Verification items for the finished model (mm, model axes). Give positions to 0.01 mm unless a question says otherwise; leave off trailing zeros. Write each loop counter-clockwise with the first axis right and the second up, starting at its lowest first coordinate (ties: lowest second). Pieces come first, ordered by that corner, then holes. Notation, with made-up numbers: (65.5, -39) - (93.5, -39) arc R31 ccw to (93.5, -1) - close; hole circle Ø2 at (-21.5, 82.5). An arc over 180 degrees is marked (long way). Put each result on its own line as item: value.
from build123d import *

# Parameters (mm, degrees)
SKETCH1_W           = 355.6
SKETCH1_H           = 406.4
BOSS_EXTRUDE1_DEPTH = 6.35
CUT_EXTRUDE1_DEPTH  = 6.35


with BuildPart() as part:
    # Sketch1 → Boss-Extrude1 (new body)
    with BuildSketch(Plane(origin=(0, 0, 0), x_dir=(1, 0, 0), z_dir=(0, 1, 0))):
        Rectangle(SKETCH1_W, SKETCH1_H)
    extrude(amount=BOSS_EXTRUDE1_DEPTH)

    # Sketch2 → Cut-Extrude1 (cut)
    with BuildSketch(Plane(origin=(0, 6.35, 0), x_dir=(1, 0, 0), z_dir=(0, 1, 0))):
        with BuildLine():
            Line((-161.8361, 152.4), (-161.8361, -152.4))
            ThreePointArc((-161.8361, -152.4), (-165.1, -155.6639), (-168.3639, -152.4))
            Line((-168.3639, -152.4), (-168.3639, 152.4))
            ThreePointArc((-168.3639, 152.4), (-165.1, 155.6639), (-161.8361, 152.4))
        make_face()
    cut_extrude1 = extrude(amount=-CUT_EXTRUDE1_DEPTH, mode=Mode.SUBTRACT)

    # Mirror1: Cut-Extrude1 across plane
    add(cut_extrude1.mirror(Plane(origin=(0, 0, 0), x_dir=(0, 0, 1), z_dir=(1, 0, 0))), mode=Mode.SUBTRACT)


solid = part.part
Q1. Section check A-A, the plane z = -47.5. Record the cut outline in (x, y), plus the area to 3 significant figures.
Answers follow:
outline: (-177.8, 0) - (-168.36, 0) - (-168.36, 6.35) - (-177.8, 6.35) - close; (-161.84, 0) - (161.84, 0) - (161.84, 6.35) - (-161.84, 6.35) - close; (168.36, 0) - (177.8, 0) - (177.8, 6.35) - (168.36, 6.35) - close
area: 2,180 mm2
Q2. Section check B-B, the plane y = 5. Record the cut outline in (x, z), plus the area to 3 significant figures.
Answers follow:
outline: (-177.8, -203.2) - (177.8, -203.2) - (177.8, 203.2) - (-177.8, 203.2) - close; hole (-168.36, -152.4) arc R3.26 ccw to (-161.84, -152.4) - (-161.84, 152.4) arc R3.26 ccw to (-168.36, 152.4) - close; hole (161.84, -152.4) arc R3.26 ccw to (168.36, -152.4) - (168.36, 152.4) arc R3.26 ccw to (161.84, 152.4) - close
area: 140,000 mm2
Q3. Scan line: line 1 along X through (y, z) = (5, -125.5). Record every from-to range of solid material in increasing order.
Answers follow:
line 1: x = -177.8 to -168.36, -161.84 to 161.84, 168.36 to 177.8
